Model file for the job. Use its own axes, mm. Round coordinates to 2 decimals unless told otherwise and drop trailing zeros. Write each loop counter-clockwise with the first axis right and the second up, starting at its lowest first coordinate (ties: lowest second). Pieces come first, ordered by that corner, then holes.
```python
from build123d import *

# Parameters (mm, degrees)
SKETCH_1_W          = 6
SKETCH_1_H          = 6
EXTRUDE_1_DEPTH     = 6
SKETCH_2_R          = 1.4
CUT_EXTRUDE_1_DEPTH = 7
CUT_EXTRUDE_2_DEPTH = 7


with BuildPart() as part:
    # ｽｹｯﾁ1 → ﾎﾞｽ - 押し出し1 (new body)
    with BuildSketch(Plane.XY):
        with Locations((0.221154353, -0.1069869)):
            Rectangle(SKETCH_1_W, SKETCH_1_H)
    extrude(amount=EXTRUDE_1_DEPTH)

    # ｽｹｯﾁ2 → ｶｯﾄ - 押し出し1 (cut, through all)
    with BuildSketch(Plane.XY.offset(6)):
        with Locations((0.221154353, -0.1069869)):
            Circle(SKETCH_2_R)
    extrude(amount=-CUT_EXTRUDE_1_DEPTH, mode=Mode.SUBTRACT)

    # ｽｹｯﾁ3 → ｶｯﾄ - 押し出し2 (cut, through all)
    with BuildSketch(Plane(origin=(3.221154353, 0, 0), x_dir=(0, 0, -1), z_dir=(1, 0, 0))):
        Polygon((-6, -3.1069869), (-6, -2.9069869), (-5.8, -3.1069869), align=None)
    extrude(amount=-CUT_EXTRUDE_2_DEPTH, mode=Mode.SUBTRACT)


solid = part.part
```
1) Cut at A-A on y = 0.05. List the corners of the cut face in (x, z).
2) Cut at B-B on x = 1.2. List the corners of the cut face in (y, z), and give its area (3 significant figures).
3) Pull direction Y, two halves, no side cores. Call faces 1 (the face through (3.221, 0, 3)), 2 (the face through (-0.082, -1.474, 3.042)), 3 (the face through (0, -3.107, 3)), 4 (the face through (0, 2.893, 3)): released by +Y, released by -Y, zero draft, split by the parting line, or undercut.
4) Cut at D-D on y = -0.75. List the corners of the cut face in (x, z).
5) Cut at C-C on z = 4.3. List the corners of the cut face in (x, y), and give its area (3 significant figures).
6) Wall check: probe 1 along Y at (x, z) = (0.3, 3.9); probe 2 along Y at (x, z) = (0.75, 3); probe 3 along X at (y, z) = (-0.3, 3.3). Give the ranges that are in metal, low to high.
7) Flat gauge pins, fed straight in: pin 1 Ø1.7 at (x, y) = (0.22, -0.11) entering from +Z; pin 2 Ø1 at (x, y) = (1, -2) entering from -Z. Where does each tip first touch, or does it go through?
Result sheet:
1. outline: (-2.78, 0) - (-1.17, 0) - (-1.17, 6) - (-2.78, 6) - close; (1.61, 0) - (3.22, 0) - (3.22, 6) - (1.61, 6) - close
2. outline: (-3.11, 0) - (-1.11, 0) - (-1.11, 6) - (-2.91, 6) - (-3.11, 5.8) - close; (0.89, 0) - (2.89, 0) - (2.89, 6) - (0.89, 6) - close
2. area: 24.0 mm2
3. face 1: zero draft
3. face 2: undercut
3. face 3: released by -Y
3. face 4: released by +Y
4. outline: (-2.78, 0) - (-1.02, 0) - (-1.02, 6) - (-2.78, 6) - close; (1.46, 0) - (3.22, 0) - (3.22, 6) - (1.46, 6) - close
5. outline: (-2.78, -3.11) - (3.22, -3.11) - (3.22, 2.89) - (-2.78, 2.89) - close; hole circle Ø2.8 at (0.22, -0.11)
5. area: 29.8 mm2
6. probe 1: y = -3.11 to -1.5, 1.29 to 2.89
6. probe 2: y = -3.11 to -1.4, 1.19 to 2.89
6. probe 3: x = -2.78 to -1.17, 1.61 to 3.22
7. pin 1: passes through
7. pin 2: stops at z = 0
